from build123d import *

# Parameters (mm, degrees)
F0_W     = 80
F0_H     = 160.5
F0_R     = 3.25
F1_DEPTH = 5


# Not quite as in the source:
# - a feature of the source that left no trace in its solid (it failed there, or was rolled back) is left out


with BuildPart() as f1:
    # F0 (on Top) → F1 (new body)
    with BuildSketch(Plane.XY):
        Rectangle(F0_W, F0_H)
        with Locations((-20, -39.75)):
            Circle(F0_R, mode=Mode.SUBTRACT)
        with Locations((-20, -29.75)):
            Circle(F0_R, mode=Mode.SUBTRACT)
        with Locations((-10, -39.75)):
            Circle(F0_R, mode=Mode.SUBTRACT)
        with Locations((-10, -29.75)):
            Circle(F0_R, mode=Mode.SUBTRACT)
        with Locations((-20, -19.75)):
            Circle(F0_R, mode=Mode.SUBTRACT)
        with Locations((-20, -9.75)):
            Circle(F0_R, mode=Mode.SUBTRACT)
        with Locations((-10, -19.75)):
            Circle(F0_R, mode=Mode.SUBTRACT)
        with Locations((-10, -9.75)):
            Circle(F0_R, mode=Mode.SUBTRACT)
        with Locations((0, -39.75)):
            Circle(F0_R, mode=Mode.SUBTRACT)
        with Locations((0, -29.75)):
            Circle(F0_R, mode=Mode.SUBTRACT)
        with Locations((10, -39.75)):
            Circle(F0_R, mode=Mode.SUBTRACT)
        with Locations((10, -29.75)):
            Circle(F0_R, mode=Mode.SUBTRACT)
        with Locations((0, -19.75)):
            Circle(F0_R, mode=Mode.SUBTRACT)
        with Locations((0, -9.75)):
            Circle(F0_R, mode=Mode.SUBTRACT)
        with Locations((10, -19.75)):
            Circle(F0_R, mode=Mode.SUBTRACT)
        with Locations((10, -9.75)):
            Circle(F0_R, mode=Mode.SUBTRACT)
        with Locations((20, -39.75)):
            Circle(F0_R, mode=Mode.SUBTRACT)
        with Locations((20, -29.75)):
            Circle(F0_R, mode=Mode.SUBTRACT)
        with Locations((20, -19.75)):
            Circle(F0_R, mode=Mode.SUBTRACT)
        with Locations((20, -9.75)):
            Circle(F0_R, mode=Mode.SUBTRACT)
        with Locations((-20, 0.25)):
            Circle(F0_R, mode=Mode.SUBTRACT)
        with Locations((-20, 10.25)):
            Circle(F0_R, mode=Mode.SUBTRACT)
        with Locations((-10, 0.25)):
            Circle(F0_R, mode=Mode.SUBTRACT)
        with Locations((-10, 10.25)):
            Circle(F0_R, mode=Mode.SUBTRACT)
        with Locations((-20, 20.25)):
            Circle(F0_R, mode=Mode.SUBTRACT)
        with Locations((-20, 30.25)):
            Circle(F0_R, mode=Mode.SUBTRACT)
        with Locations((-10, 20.25)):
            Circle(F0_R, mode=Mode.SUBTRACT)
        with Locations((-10, 30.25)):
            Circle(F0_R, mode=Mode.SUBTRACT)
        with Locations((-20, 40.25)):
            Circle(F0_R, mode=Mode.SUBTRACT)
        with Locations((-10, 40.25)):
            Circle(F0_R, mode=Mode.SUBTRACT)
        with Locations((0, 0.25)):
            Circle(F0_R, mode=Mode.SUBTRACT)
        with Locations((0, 10.25)):
            Circle(F0_R, mode=Mode.SUBTRACT)
        with Locations((10, 0.25)):
            Circle(F0_R, mode=Mode.SUBTRACT)
        with Locations((10, 10.25)):
            Circle(F0_R, mode=Mode.SUBTRACT)
        with Locations((0, 20.25)):
            Circle(F0_R, mode=Mode.SUBTRACT)
        with Locations((0, 30.25)):
            Circle(F0_R, mode=Mode.SUBTRACT)
        with Locations((10, 20.25)):
            Circle(F0_R, mode=Mode.SUBTRACT)
        with Locations((10, 30.25)):
            Circle(F0_R, mode=Mode.SUBTRACT)
        with Locations((20, 0.25)):
            Circle(F0_R, mode=Mode.SUBTRACT)
        with Locations((20, 10.25)):
            Circle(F0_R, mode=Mode.SUBTRACT)
        with Locations((20, 20.25)):
            Circle(F0_R, mode=Mode.SUBTRACT)
        with Locations((20, 30.25)):
            Circle(F0_R, mode=Mode.SUBTRACT)
        with Locations((0, 40.25)):
            Circle(F0_R, mode=Mode.SUBTRACT)
        with Locations((10, 40.25)):
            Circle(F0_R, mode=Mode.SUBTRACT)
        with Locations((20, 40.25)):
            Circle(F0_R, mode=Mode.SUBTRACT)
    extrude(amount=F1_DEPTH)


solid = f1.part
Work out the finished part from the listing and answer in its coordinate system (mm). Coordinates: 2 decimals unless noted, no trailing zeros. Loops run counter-clockwise (first coordinate to the right, second up) from the corner with the lowest first, then second, coordinate; pieces in that order, holes last. Notation, with made-up numbers: (25.5, -40) -> (76.5, -40) arc R14 ccw to (76.5, -22) -> close; hole circle Ø5 at (-3, 42). An arc over 180 degrees is marked (long way). Write each question's results on one line, items separated by ' | '. Start each with the question number.
1) The mould has two halves that part along X. Classify faces 1 (the cylindrical face through (-0.423, -16.528, 2.465)), 2 (the flat face through (-1, -80.25, 2)): pulls with the +X half, pulls with the -X half, needs draft (parallel to the pull), parting line crosses it, or undercut.
2) Find section B-B on x = 20. Count the separate pieces of the cut face and the enclosed holes in it, then the cut area to 3 significant figures.
3) Consider line 1 along X through (y, z) = (42, 4.6). Determine where the line is inside the solid, lowest interval first.
4) Find section A-A on y = 40.25. Determine the outline of the cut face in (x, z).
Response values:
1) face 1: undercut | face 2: needs draft
2) separate pieces: 10 | enclosed holes: 0 | area: 510 mm^2
3) line 1: x = -40 to -22.74, -17.26 to -12.74, -7.26 to -2.74, 2.74 to 7.26, 12.74 to 17.26, 22.74 to 40
4) outline: (-40, 0) -> (-23.25, 0) -> (-23.25, 5) -> (-40, 5) -> close; (-16.75, 0) -> (-13.25, 0) -> (-13.25, 5) -> (-16.75, 5) -> close; (-6.75, 0) -> (-3.25, 0) -> (-3.25, 5) -> (-6.75, 5) -> close; (3.25, 0) -> (6.75, 0) -> (6.75, 5) -> (3.25, 5) -> close; (13.25, 0) -> (16.75, 0) -> (16.75, 5) -> (13.25, 5) -> close; (23.25, 0) -> (40, 0) -> (40, 5) -> (23.25, 5) -> close
